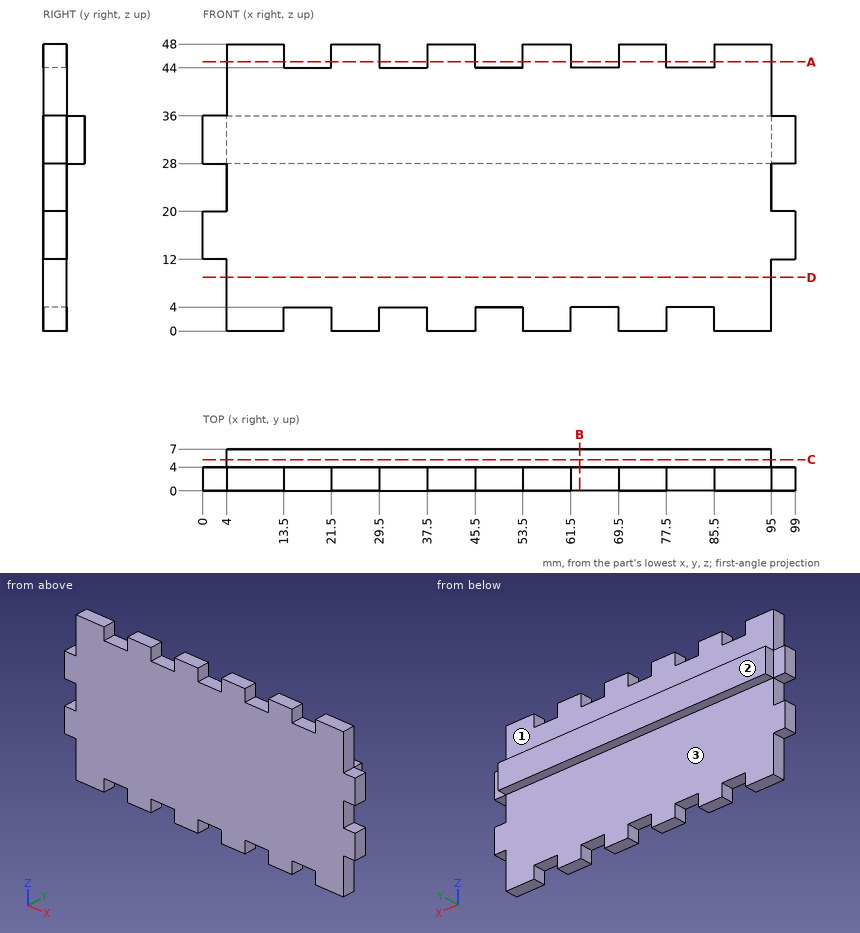
Can you work these out from the drawing? Everything is in mm from the part's minimum corner. A direction names the side the tool comes from. Round coordinates to 2 decimals unless told otherwise and drop trailing zeros. Order: outer loops, then holes, each group sorted by start corner. A loop starts at its lowest first (then second) coordinate and runs counter-clockwise, first axis right, second up.
(1) If I drill on L1, parallel to Y at x = 13.5, z = 4.5; L2, parallel to Z at x = 47.5, y = 4.5; L3, parallel to X at y = 2.25, z = 7, over which ranges is the centre line in solid material (lowest first)?
Results are:
L1: y = 0 to 4
L2: z = 28 to 36
L3: x = 4 to 95
(2) I'm going to push flat-ended pins straight in: pin 1 (3 mm diameter, centred on y = 1.5, z = 45.5, fed in from -X); pin 2 (3.5 mm diameter, centred on x = 66.5, y = 5.5, fed in from +Z); pin 3 (1 mm diameter, centred on x = 51.5, y = 6, fed in from -Z). Where does each tip first touch, or does it pass through?
Results are:
pin 1: stops at x = 4
pin 2: stops at z = 44
pin 3: stops at z = 28
(3) If we section it at A-A (z = 45): Please give me the cut outline in (x, y), plus the area to 3 significant figures.
Results are:
outline: (4, 0) - (13.5, 0) - (13.5, 4) - (4, 4) - close; (21.5, 0) - (29.5, 0) - (29.5, 4) - (21.5, 4) - close; (37.5, 0) - (45.5, 0) - (45.5, 4) - (37.5, 4) - close; (53.5, 0) - (61.5, 0) - (61.5, 4) - (53.5, 4) - close; (69.5, 0) - (77.5, 0) - (77.5, 4) - (69.5, 4) - close; (85.5, 0) - (95, 0) - (95, 4) - (85.5, 4) - close
area: 204 mm2
(4) On a 3-axis mill with a long thin cutter (end or side, diameter ignored), from which of +Z, -Z, +X, -X, +Y, -Y can I reach the whole of each face in a straight line? I mean the marked faces 1, 2 and 3. Say none if no direction works.
Results are:
face 1: +Z, +X, -X, +Y
face 2: +Z, -Z, +X, -X, +Y
face 3: -Z, +X, -X, +Y
(5) If we section it at C-C (y = 5.25): Please give me the cut outline in (x, z).
Results are:
outline: (4, 28) - (95, 28) - (95, 36) - (4, 36) - close
(6) If we section it at B-B (x = 63): Please give me the cut outline in (y, z), plus the area to 3 significant figures.
Results are:
outline: (0, 4) - (4, 4) - (4, 28) - (7, 28) - (7, 36) - (4, 36) - (4, 44) - (0, 44) - close
area: 184 mm2
(7) If we section it at D-D (z = 9): Please give me the cut outline in (x, y), plus the area to 3 significant figures.
Results are:
outline: (4, 0) - (95, 0) - (95, 4) - (4, 4) - close
area: 364 mm2
